For this review, take the finished solid that the model builds, in its own axes (mm). Round coordinates to 2 decimals unless told otherwise and drop trailing zeros. Order: outer loops, then holes, each group sorted by start corner. A loop starts at its lowest first (then second) coordinate and runs counter-clockwise, first axis right, second up. Notation, with made-up numbers: (61.25, -10) -> (103.25, -10) arc R23 cw to (103.25, 20) -> close; hole circle Ø2 at (17.25, 74.5). An arc over 180 degrees is marked (long way). Answer in a Markdown table with one row per item.
```python
from build123d import *

# Parameters (mm, degrees)
SKETCH1_R           = 2.0701
BOSS_EXTRUDE1_DEPTH = 2.286


with BuildPart() as part:
    # Sketch1 → Boss-Extrude1 (new body)
    with BuildSketch(Plane.XY.offset(2.286)):
        with BuildLine():
            Line((57.023, 10.541), (54.864, 12.7))
            Line((54.864, 12.7), (19.05, 12.7))
            ThreePointArc((19.05, 12.7), (14.559871939, 14.559871939), (12.7, 19.05))
            Line((12.7, 19.05), (12.7, 54.864))
            Line((12.7, 54.864), (10.541, 57.023))
            Line((10.541, 57.023), (-10.541, 57.023))
            Line((-10.541, 57.023), (-12.7, 54.864))
            Line((-12.7, 54.864), (-12.7, 19.05))
            ThreePointArc((-12.7, 19.05), (-14.559871939, 14.559871939), (-19.05, 12.7))
            Line((-19.05, 12.7), (-54.864, 12.7))
            Line((-54.864, 12.7), (-57.023, 10.541))
            Line((-57.023, 10.541), (-57.023, -10.541))
            Line((-57.023, -10.541), (-54.864, -12.7))
            Line((-54.864, -12.7), (-19.05, -12.7))
            ThreePointArc((-19.05, -12.7), (-14.559871939, -14.559871939), (-12.7, -19.05))
            Line((-12.7, -19.05), (-12.7, -54.864))
            Line((-12.7, -54.864), (-10.541, -57.023))
            Line((-10.541, -57.023), (10.541, -57.023))
            Line((10.541, -57.023), (12.7, -54.864))
            Line((12.7, -54.864), (12.7, -19.05))
            ThreePointArc((12.7, -19.05), (14.559871939, -14.559871939), (19.05, -12.7))
            Line((19.05, -12.7), (54.864, -12.7))
            Line((54.864, -12.7), (57.023, -10.541))
            Line((57.023, -10.541), (57.023, 10.541))
        make_face()
        with Locations((0, 12.7)):
            Circle(SKETCH1_R, mode=Mode.SUBTRACT)
        with Locations((0, 38.1)):
            Circle(SKETCH1_R, mode=Mode.SUBTRACT)
        with Locations((-12.7, 0)):
            Circle(SKETCH1_R, mode=Mode.SUBTRACT)
        with Locations((-38.1, 0)):
            Circle(SKETCH1_R, mode=Mode.SUBTRACT)
        with Locations((50.8, 0)):
            Circle(SKETCH1_R, mode=Mode.SUBTRACT)
        with Locations((0, -38.1)):
            Circle(SKETCH1_R, mode=Mode.SUBTRACT)
        with Locations((0, -12.7)):
            Circle(SKETCH1_R, mode=Mode.SUBTRACT)
        with Locations((25.4, 0)):
            Circle(SKETCH1_R, mode=Mode.SUBTRACT)
        Circle(SKETCH1_R, mode=Mode.SUBTRACT)
        with Locations((12.7, 0)):
            Circle(SKETCH1_R, mode=Mode.SUBTRACT)
        with Locations((38.1, 0)):
            Circle(SKETCH1_R, mode=Mode.SUBTRACT)
        with Locations((0, -25.4)):
            Circle(SKETCH1_R, mode=Mode.SUBTRACT)
        with Locations((0, -50.8)):
            Circle(SKETCH1_R, mode=Mode.SUBTRACT)
        with Locations((-50.8, 0)):
            Circle(SKETCH1_R, mode=Mode.SUBTRACT)
        with Locations((-25.4, 0)):
            Circle(SKETCH1_R, mode=Mode.SUBTRACT)
        with Locations((0, 50.8)):
            Circle(SKETCH1_R, mode=Mode.SUBTRACT)
        with Locations((0, 25.4)):
            Circle(SKETCH1_R, mode=Mode.SUBTRACT)
    extrude(amount=-BOSS_EXTRUDE1_DEPTH)


solid = part.part
```
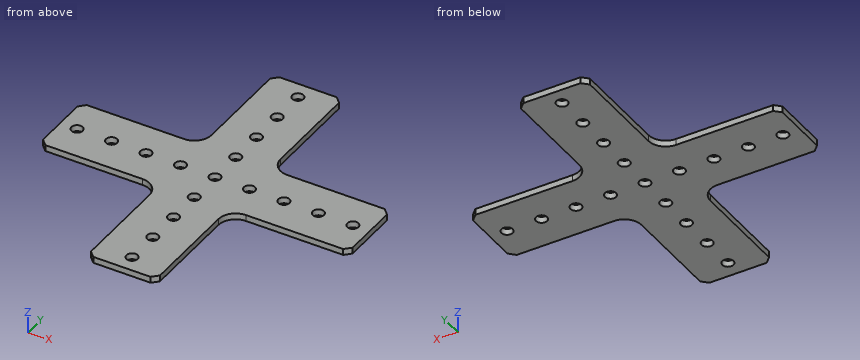
Q1. Take a section at A-A, the plane y = 25.4. Write out the cut boundary in (x, z).
Answer key:
| item | result |
|---|---|
| outline | (-12.7, 0) -> (-2.07, 0) -> (-2.07, 2.29) -> (-12.7, 2.29) -> close; (2.07, 0) -> (12.7, 0) -> (12.7, 2.29) -> (2.07, 2.29) -> close |
Q2. Clearance check with flat-ended pins moving along their axes: pin 1 Ø0.7 at (y, z) = (41.5, 0.5) entering from +X; pin 2 Ø1 at (y, z) = (35, 1) entering from -X; pin 3 Ø1.1 at (x, z) = (-32, 0.5) entering from -Y. State where each tip first meets the part, or that it passes through.
Answer key:
| item | result |
|---|---|
| pin 1 | stops at x = 12.7 |
| pin 2 | stops at x = -12.7 |
| pin 3 | stops at y = -12.7 |
Q3. Take a section at C-C, the plane x = 0. Give the number of separate pieces and of enclosed holes in the cut face, then the cut area to 3 significant figures.
Answer key:
| item | result |
|---|---|
| separate pieces | 10 |
| enclosed holes | 0 |
| area | 176 mm^2 |
Q4. To check wall thickness, follow probe 1 along Y at (x, z) = (-50.8, 0.65); probe 2 along X at (y, z) = (40.5, 1.3). State the ranges of each line that lie inside material, in increasing order.
Answer key:
| item | result |
|---|---|
| probe 1 | y = -12.7 to -2.07, 2.07 to 12.7 |
| probe 2 | x = -12.7 to 12.7 |
